Could you check a few things on this model? Use its own coordinates, in mm. Face numbers are marked on the shaded views. A direction names the side the tool comes from. Coordinates: 2 decimals unless noted, no trailing zeros. Order: outer loops, then holes, each group sorted by start corner. A loop starts at its lowest first (then second) coordinate and runs counter-clockwise, first axis right, second up. Notation, with made-up numbers: (86.5, 16.25) -> (96.5, 16.25) arc R28 ccw to (96.5, 44.25) -> close; hole circle Ø7 at (59.25, 4.25). An arc over 180 degrees is marked (long way). Put each result on its own line as item: value. Start each with the question number.
Q1. Please list where these lines run through material, in increasing order: line 1 along X through (y, z) = (29.95, -70); line 2 along X through (y, z) = (30.25, -78); line 3 along Y through (x, z) = (-13, -9).
Q2. If we section it at C-C (x = -7.5): Please give me the cut outline in (y, z), and give its area (3 significant figures).
Q3. If we section it at B-B (y = 30): Please give me the cut outline in (x, z), and give its area (3 significant figures).
Q4. For the marked faces 1 and 2, which set-ups out of +Z, -Z, +X, -X, +Y, -Y let a thin tool reach every point of the face, with its end or its side?
Q5. Will these pins go through, and if not, where does the flat tip stop? pin 1 (10 mm diameter, centred on x = 0, z = -78, fed in from -Y); pin 2 (1.6 mm diameter, centred on x = -14, y = 28, fed in from -Z); pin 3 (5.5 mm diameter, centred on x = 0, z = -78, fed in from +Y).
Q6. If we section it at A-A (z = -70): Please give me the cut outline in (x, y).
Q7. If we section it at D-D (z = -31.5): Please give me the cut outline in (x, y), and give its area (3 significant figures).
from build123d import *

# Parameters (mm, degrees)
BOSS_EXTRUDE1_DEPTH = 83
SKETCH3_W           = 58
SKETCH3_H           = 2
BOSS_EXTRUDE2_DEPTH = 2
FILLET1_R           = 3
SKETCH4_W           = 56.032437302
SKETCH4_H           = 2
BOSS_EXTRUDE3_DEPTH = 0.25
FILLET2_R           = 0.5
CUT_EXTRUDE1_REACH  = 91.909
SKETCH5_R           = 3
CUT_EXTRUDE2_REACH  = 91.909
SKETCH7_R           = 2
FILLET3_R           = 0.5
SKETCH8_R           = 3.75
CUT_EXTRUDE3_DEPTH  = 3


with BuildPart() as part:
    # Sketch1 → Boss-Extrude1 (new body)
    with BuildSketch(Plane.XY):
        Polygon((-26.755845082, 29), (-28.016218651, 27.2), (28.016218651, 27.2), (26.755845082, 29), (26.755845082, 29.15), (29, 29.15), (29, 31.15), (-29, 31.15), (-29, 29.15), (-26.755845082, 29.15), align=None)
    extrude(amount=-BOSS_EXTRUDE1_DEPTH)

    # Sketch3 → Boss-Extrude2 (add)
    with BuildSketch(Plane(origin=(0, 0, -83), x_dir=(-1, 0, 0), z_dir=(0, 0, -1))):
        with Locations((0, 30.15)):
            Rectangle(SKETCH3_W, SKETCH3_H)
    extrude(amount=BOSS_EXTRUDE2_DEPTH)

    # Fillet1
    fillet1_edges = [part.edges().sort_by_distance(p)[0] for p in [
        (-29, 30.15, -85),
        (29, 30.15, -85),
    ]]
    fillet(fillet1_edges, radius=FILLET1_R)

    # Sketch4 → Boss-Extrude3 (add)
    with BuildSketch(Plane.XZ.offset(-27.2)):
        with Locations((0, -2.5)):
            Rectangle(SKETCH4_W, SKETCH4_H)
    extrude(amount=BOSS_EXTRUDE3_DEPTH)

    # Fillet2
    # the kernel refuses this fillet: 0.5 mm, written as the material it takes off along each edge
    with BuildSketch(Plane(origin=(-29.098750406, 26.95, -3.5), x_dir=(0, 1, 0), z_dir=(1, 0, 0)), Plane(origin=(29.098750406, 26.95, -1.5), x_dir=(0, 1, 0), z_dir=(-1, 0, 0))) as fillet2_piece_1:
        with BuildLine():
            CenterArc((0.5, 0.433012702), FILLET2_R, 180, 60)
            Line((0, 0.433012702), (-0.01, 0.433012702))
            Line((-0.01, 0.433012702), (-0.01, 0))
            Line((-0.01, 0), (0, -0.01))
            ThreePointArc((0, -0.01), (0.125, -0.01), (0.245, -0.008660254))
            Line((0.245, -0.008660254), (0.25, 0))
        make_face()
    extrude(amount=58.197500812, mode=Mode.SUBTRACT)

    # Sketch5 → Cut-Extrude1 (cut, up to next)
    with BuildSketch(Plane(origin=(0, 31.15, 0), x_dir=(1, 0, 0), z_dir=(0, 1, 0)), mode=Mode.PRIVATE) as cut_extrude1_sk1:
        with Locations(Location((0, 78, 0), (0, 0, 270))):
            Circle(SKETCH5_R)
    cut_extrude1_tool1 = extrude(cut_extrude1_sk1.sketch, amount=-CUT_EXTRUDE1_REACH, mode=Mode.PRIVATE) & part.part
    add(cut_extrude1_tool1.solids().sort_by_distance((0, 31.15, -78))[0], mode=Mode.SUBTRACT)

    # Sketch7 → Cut-Extrude2 (cut, up to next)
    with BuildSketch(Plane(origin=(0, 31.15, 0), x_dir=(1, 0, 0), z_dir=(0, 1, 0)), mode=Mode.PRIVATE) as cut_extrude2_sk1:
        with Locations(Location((14, 15, 0), (0, 0, 270))):
            Circle(SKETCH7_R)
    cut_extrude2_tool1 = extrude(cut_extrude2_sk1.sketch, amount=-CUT_EXTRUDE2_REACH, mode=Mode.PRIVATE) & part.part
    # Sketch7 → Cut-Extrude2 (cut, up to next)
    with BuildSketch(Plane(origin=(0, 31.15, 0), x_dir=(1, 0, 0), z_dir=(0, 1, 0)), mode=Mode.PRIVATE) as cut_extrude2_sk2:
        with Locations((14, 70)):
            Circle(SKETCH7_R)
    cut_extrude2_tool2 = extrude(cut_extrude2_sk2.sketch, amount=-CUT_EXTRUDE2_REACH, mode=Mode.PRIVATE) & part.part
    # Sketch7 → Cut-Extrude2 (cut, up to next)
    with BuildSketch(Plane(origin=(0, 31.15, 0), x_dir=(1, 0, 0), z_dir=(0, 1, 0)), mode=Mode.PRIVATE) as cut_extrude2_sk3:
        with Locations(Location((-14, 70, 0), (0, 0, 270))):
            Circle(SKETCH7_R)
    cut_extrude2_tool3 = extrude(cut_extrude2_sk3.sketch, amount=-CUT_EXTRUDE2_REACH, mode=Mode.PRIVATE) & part.part
    # Sketch7 → Cut-Extrude2 (cut, up to next)
    with BuildSketch(Plane(origin=(0, 31.15, 0), x_dir=(1, 0, 0), z_dir=(0, 1, 0)), mode=Mode.PRIVATE) as cut_extrude2_sk4:
        with Locations((-14, 15)):
            Circle(SKETCH7_R)
    cut_extrude2_tool4 = extrude(cut_extrude2_sk4.sketch, amount=-CUT_EXTRUDE2_REACH, mode=Mode.PRIVATE) & part.part
    add(cut_extrude2_tool1.solids().sort_by_distance((14, 31.15, -15))[0], mode=Mode.SUBTRACT)
    add(cut_extrude2_tool2.solids().sort_by_distance((14, 31.15, -70))[0], mode=Mode.SUBTRACT)
    add(cut_extrude2_tool3.solids().sort_by_distance((-14, 31.15, -70))[0], mode=Mode.SUBTRACT)
    add(cut_extrude2_tool4.solids().sort_by_distance((-14, 31.15, -15))[0], mode=Mode.SUBTRACT)

    # Fillet3
    fillet3_edges = [part.edges().sort_by_distance(p)[0] for p in [
        (29, 31.15, -41),
        (0, 31.15, -85),
        (-29, 31.15, -41),
        (-28.121320344, 31.15, -84.121320344),
        (28.121320344, 31.15, -84.121320344),
    ]]
    fillet(fillet3_edges, radius=FILLET3_R)

    # Sketch8 → Cut-Extrude3 (cut)
    with BuildSketch(Plane(origin=(0, 31.15, 0), x_dir=(1, 0, 0), z_dir=(0, 1, 0))):
        with Locations(Location((0, 78, 0), (0, 0, 270))):
            Circle(SKETCH8_R)
    extrude(amount=-CUT_EXTRUDE3_DEPTH, mode=Mode.SUBTRACT)


solid = part.part
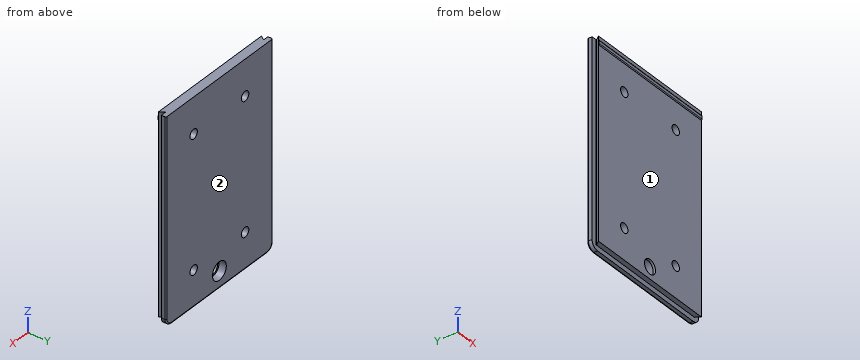
The answers:
1. line 1: -29 to -16, -12 to 12, 16 to 29
1. line 2: -29 to -3.75, 3.75 to 29
1. line 3: 27.2 to 31.15
2. outline: (26.95, -3.07) arc R0.5 ccw to (27.2, -3.5) -> (27.2, -83) -> (29.15, -83) -> (29.15, -85) -> (30.65, -85) arc R0.5 ccw to (31.15, -84.5) -> (31.15, 0) -> (27.2, 0) -> (27.2, -1.5) arc R0.5 ccw to (26.95, -1.93) -> close
2. area: 332 mm^2
3. outline: (-29, -82) arc R3 ccw to (-26, -85) -> (26, -85) arc R3 ccw to (29, -82) -> (29, 0) -> (-29, 0) -> close; hole circle Ø4 at (-14, -70); hole circle Ø4 at (-14, -15); hole circle Ø7.5 at (0, -78); hole circle Ø4 at (14, -70); hole circle Ø4 at (14, -15)
3. area: 4,830 mm^2
4. face 1: -Z, +X, -X, -Y
4. face 2: +Z, -Z, +X, -X, +Y
5. pin 1: y = 27.2
5. pin 2: z = -83
5. pin 3: through
6. outline: (-29, 29.15) -> (-26.76, 29.15) -> (-26.76, 29) -> (-28.02, 27.2) -> (-16, 27.2) -> (-16, 31.15) -> (-28.5, 31.15) arc R0.5 ccw to (-29, 30.65) -> close; (-12, 27.2) -> (12, 27.2) -> (12, 31.15) -> (-12, 31.15) -> close; (16, 27.2) -> (28.02, 27.2) -> (26.76, 29) -> (26.76, 29.15) -> (29, 29.15) -> (29, 30.65) arc R0.5 ccw to (28.5, 31.15) -> (16, 31.15) -> close
7. outline: (-29, 29.15) -> (-26.76, 29.15) -> (-26.76, 29) -> (-28.02, 27.2) -> (28.02, 27.2) -> (26.76, 29) -> (26.76, 29.15) -> (29, 29.15) -> (29, 30.65) arc R0.5 ccw to (28.5, 31.15) -> (-28.5, 31.15) arc R0.5 ccw to (-29, 30.65) -> close
7. area: 223 mm^2
